For this review, take the finished solid that the model builds, in its own axes (mm). Face numbers are marked on the shaded views. A direction names the side the tool comes from. Coordinates: 2 decimals unless noted, no trailing zeros. Order: outer loops, then holes, each group sorted by start corner. A loop starts at its lowest first (then second) coordinate and runs counter-clockwise, first axis right, second up.
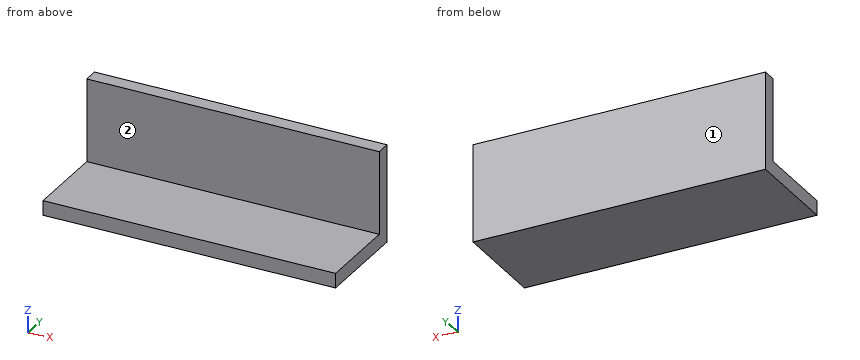
from build123d import *

# Parameters (mm, degrees)
F0_W     = 30
F0_H     = 1.5
F0_H_2   = 8.5
F1_DEPTH = 1.5
F2_DEPTH = 10


with BuildPart() as f1:
    # F0 (on Top) → F1 (new body)
    with BuildSketch(Plane.XY):
        with Locations((6.926514, 0.62533)):
            Rectangle(F0_W, F0_H)
        with Locations((6.926514, -4.37467)):
            Rectangle(F0_W, F0_H_2)
    extrude(amount=F1_DEPTH)

    # F0 (on Top) → F2 (join)
    with BuildSketch(Plane.XY):
        with Locations((6.926514, 0.62533)):
            Rectangle(F0_W, F0_H)
    extrude(amount=F2_DEPTH)


solid = f1.part
1. Take a section at C-C, the plane y = -1.75. Give the boundary of the cut face in (x, z), plus the area to 3 significant figures.
Answer below:
outline: (-8.07, 0) - (21.93, 0) - (21.93, 1.5) - (-8.07, 1.5) - close
area: 45.0 mm2
2. To check wall thickness, follow L1, parallel to Z at x = 17, y = -2; L2, parallel to Y at x = -4, z = 2.5. State the ranges of each line that lie inside material, in increasing order.
Answer below:
L1: z = 0 to 1.5
L2: y = -0.12 to 1.38
3. Take a section at B-B, the plane z = 7. Give the boundary of the cut face in (x, y), plus the area to 3 significant figures.
Answer below:
outline: (-8.07, -0.12) - (21.93, -0.12) - (21.93, 1.38) - (-8.07, 1.38) - close
area: 45.0 mm2
4. Clearance check with flat-ended pins moving along their axes: pin 1 Ø5 at (x, y) = (-3, -4.5) entering from +Z; pin 2 Ø2.5 at (x, z) = (12, 6) entering from -Y; pin 3 Ø1.5 at (y, z) = (-4.5, 2) entering from -X. State where each tip first meets the part, or that it passes through.
Answer below:
pin 1: stops at z = 1.5
pin 2: stops at y = -0.12
pin 3: stops at x = -8.07
5. Take a section at A-A, the plane x = 12. Give the boundary of the cut face in (y, z), plus the area to 4 significant figures.
Answer below:
outline: (-8.62, 0) - (1.38, 0) - (1.38, 10) - (-0.12, 10) - (-0.12, 1.5) - (-8.62, 1.5) - close
area: 27.75 mm2
6. Machinability: for the marked faces 1 and 2, which of the approach directions +Z, -Z, +X, -X, +Y, -Y give a long, thin tool a straight path to every point of the face, cutting with its end or side? Answer none if there is none.
Answer below:
face 1: +Z, -Z, +X, -X, +Y
face 2: +Z, +X, -X, -Y
